```python
from build123d import *

# Parameters (mm, degrees)
SKETCH_R  = 2.5
PAD_DEPTH = 6


with BuildPart() as part:
    # Sketch → Pad (new body)
    with BuildSketch(Plane.XY):
        with BuildLine():
            Line((181.480679, 0), (181.480679, 63.633531))
            Line((181.480679, 63.633531), (100, 180))
            Line((100, 180), (0, 180))
            Line((0, 180), (0, 100))
            Line((0, 100), (60, 100))
            ThreePointArc((111.77515, 48.22485), (96.61056, 84.83541), (60, 100))
            Line((111.77515, 48.22485), (111.77515, 0))
            Line((111.77515, 0), (181.480679, 0))
        make_face()
        with Locations((10, 170)):
            Circle(SKETCH_R, mode=Mode.SUBTRACT)
        with Locations((30, 170)):
            Circle(SKETCH_R, mode=Mode.SUBTRACT)
        with Locations((30, 150)):
            Circle(SKETCH_R, mode=Mode.SUBTRACT)
        with Locations((30, 130)):
            Circle(SKETCH_R, mode=Mode.SUBTRACT)
        with Locations((30, 110)):
            Circle(SKETCH_R, mode=Mode.SUBTRACT)
        with Locations((10, 110)):
            Circle(SKETCH_R, mode=Mode.SUBTRACT)
    extrude(amount=PAD_DEPTH)


solid = part.part
```
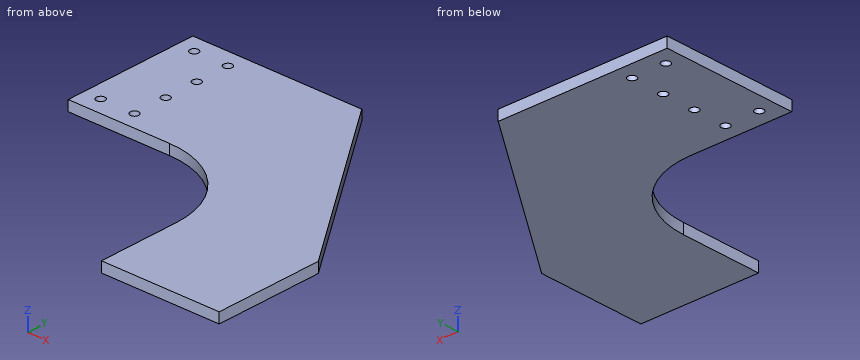
Check sheet for the modelled part. Datum: model origin and axes. Units: mm. Round coordinates to 2 decimals unless told otherwise and drop trailing zeros. Write each loop counter-clockwise with the first axis right and the second up, starting at its lowest first coordinate (ties: lowest second). Pieces come first, ordered by that corner, then holes. Notation, with made-up numbers: (-34, 43.25) -> (0, 43.25) arc R16 cw to (0, 51.25) -> close; hole circle Ø2 at (69, 76.25). An arc over 180 degrees is marked (long way). Put each result on its own line as item: value.
(1) Sectioned sample at A-A (y = 150). Enter the section's corners in (x, z).
Values found:
outline: (0, 0) -> (27.5, 0) -> (27.5, 6) -> (0, 6) -> close; (32.5, 0) -> (121.01, 0) -> (121.01, 6) -> (32.5, 6) -> close
(2) Sectioned sample at B-B (z = 4.65). Enter the section's corners in (x, y).
Values found:
outline: (0, 100) -> (60, 100) arc R51.78 cw to (111.78, 48.22) -> (111.78, 0) -> (181.48, 0) -> (181.48, 63.63) -> (100, 180) -> (0, 180) -> close; hole circle Ø5 at (10, 110); hole circle Ø5 at (10, 170); hole circle Ø5 at (30, 110); hole circle Ø5 at (30, 130); hole circle Ø5 at (30, 150); hole circle Ø5 at (30, 170)
(3) Sectioned sample at C-C (y = 110). Enter the section's corners in (x, z), plus the area to 3 significant figures.
Values found:
outline: (0, 0) -> (7.5, 0) -> (7.5, 6) -> (0, 6) -> close; (12.5, 0) -> (27.5, 0) -> (27.5, 6) -> (12.5, 6) -> close; (32.5, 0) -> (149.01, 0) -> (149.01, 6) -> (32.5, 6) -> close
area: 834 mm^2
(4) Sectioned sample at D-D (x = 25). Enter the section's corners in (y, z), plus the area to 3 significant figures.
Values found:
outline: (100, 0) -> (180, 0) -> (180, 6) -> (100, 6) -> close
area: 480 mm^2
(5) Go/stop test with a flat-tipped pin: pin 1 Ø8 at (x, y) = (10, 170) entering from -Z. Record where the tip stops, or that it passes through.
Values found:
pin 1: stops at z = 0
(6) Material ranges on line 1 (Y direction, x = 30, z = 4.35); line 2 (Y direction, x = 10, z = 1.35); line 3 (X direction, y = 168, z = 3), recorded low to high.
Values found:
line 1: y = 100 to 107.5, 112.5 to 127.5, 132.5 to 147.5, 152.5 to 167.5, 172.5 to 180
line 2: y = 100 to 107.5, 112.5 to 167.5, 172.5 to 180
line 3: x = 0 to 8.5, 11.5 to 28.5, 31.5 to 108.4
